Source: CAD feature listing. Evaluate the final solid. Frame: model axes, mm. A direction names the side the tool comes from. Give positions to 0.01 mm unless a question says otherwise; leave off trailing zeros. Write each loop counter-clockwise with the first axis right and the second up, starting at its lowest first coordinate (ties: lowest second). Pieces come first, ordered by that corner, then holes. Notation, with made-up numbers: (50.25, 17.25) -> (102.25, 17.25) arc R29 cw to (102.25, 51.25) -> close; hole circle Ø5 at (-13.5, 78). An arc over 180 degrees is marked (long way). Write item = value, one per line.
from build123d import *

# Parameters (mm, degrees)
BOSS_EXTRUDE1_DEPTH = 127
CUT_EXTRUDE1_REACH  = 39.846
SKETCH3_R           = 6.35


with BuildPart() as part:
    # Sketch1 → Boss-Extrude1 (new body, symmetric)
    with BuildSketch(Plane.XY):
        with BuildLine():
            Line((37.846, -38.1), (0, -38.1))
            Line((0, -38.1), (0, 38.1))
            Line((0, 38.1), (37.846, 38.1))
            Line((37.846, 38.1), (37.846, 38.095373852))
            Line((37.846, 38.095373852), (37.846, 38.07919906))
            ThreePointArc((37.846, 38.07919906), (37.304749426, 36.602159643), (35.937298827, 35.824550175))
            Line((35.937298827, 35.824550175), (12.279303519, 31.865559515))
            ThreePointArc((12.279303519, 31.865559515), (8.176951722, 29.532731112), (6.5532, 25.101612859))
            Line((6.5532, 25.101612859), (6.5532, -24.125928831))
            ThreePointArc((6.5532, -24.125928831), (8.176951722, -28.557047083), (12.279303519, -30.889875486))
            Line((12.279303519, -30.889875486), (35.725220919, -34.813376476))
            ThreePointArc((35.725220919, -34.813376476), (37.244610473, -35.677386996), (37.846, -37.318541904))
            Line((37.846, -37.318541904), (37.846, -38.1))
        make_face()
    extrude(amount=BOSS_EXTRUDE1_DEPTH, both=True)

    # Sketch3 → Cut-Extrude1 (cut, up to next)
    with BuildSketch(Plane.ZY, mode=Mode.PRIVATE) as cut_extrude1_sk1:
        with Locations((-15.875, 0)):
            Circle(SKETCH3_R)
    cut_extrude1_tool1 = extrude(cut_extrude1_sk1.sketch, amount=-CUT_EXTRUDE1_REACH, mode=Mode.PRIVATE) & part.part
    add(cut_extrude1_tool1.solids().sort_by_distance((0, 0, -15.875))[0], mode=Mode.SUBTRACT)
    # Sketch3 → Cut-Extrude1 (cut, up to next)
    with BuildSketch(Plane.ZY, mode=Mode.PRIVATE) as cut_extrude1_sk2:
        with Locations((15.875, 0)):
            Circle(SKETCH3_R)
    cut_extrude1_tool2 = extrude(cut_extrude1_sk2.sketch, amount=-CUT_EXTRUDE1_REACH, mode=Mode.PRIVATE) & part.part
    add(cut_extrude1_tool2.solids().sort_by_distance((0, 0, 15.875))[0], mode=Mode.SUBTRACT)


solid = part.part
1) Material intervals for L1, parallel to X at y = 1, z = 88.5; L2, parallel to Z at x = 2.5, y = -1.5; L3, parallel to Y at x = 24, z = 27.5, sorted ascending.
Computed:
L1 = 0 to 6.55
L2 = -127 to -22.05, -9.7 to 9.7, 22.05 to 127
L3 = -38.1 to -32.85, 33.83 to 38.1
2) Contact query for flat-ended pins moving along their axis: pin 1 (3 mm diameter, centred on y = 5.5, z = -10.5, fed in from -X); pin 2 (16.5 mm diameter, centred on y = 0, z = 15.875, fed in from +X). Output: stop coordinate, or through.
Computed:
pin_1 = 0
pin_2 = 6.55
3) Access query for faces 1 (the flat face through (0, -1, 2)), 2 (the flat face through (23.838, -32.824, 1.778)). Directions: +Z, -Z, +X, -X, +Y, -Y. A direction counts if a zero-diameter tool reaches every point of the face in a straight line with its end or side. Return the directions, or none.
Computed:
face_1 = +Z, -Z, -X, +Y, -Y
face_2 = +Z, -Z, +X
4) Cut plane A-A (y = 0). Return the cut outline in (x, z) (3 decimals).
Computed:
outline = (0, -127) -> (6.553, -127) -> (6.553, -22.225) -> (0, -22.225) -> close; (0, -9.525) -> (6.553, -9.525) -> (6.553, 9.525) -> (0, 9.525) -> close; (0, 22.225) -> (6.553, 22.225) -> (6.553, 127) -> (0, 127) -> close
5) Cut plane D-D (y = -15). Return the cut outline in (x, z), then the cut area to 3 significant figures.
Computed:
outline = (0, -127) -> (6.55, -127) -> (6.55, 127) -> (0, 127) -> close
area = 1,660 mm²
6) Draft query along Z for faces 3 (the cylindrical face through (3.23, 1.91, 21.93)), 4 (the flat face through (19, 38.1, 2)), 5 (the flat face through (6, 3, -127)). Return one class per face: pulls with the +Z half, pulls with the -Z half, needs draft (parallel to the pull), parting line crosses it, or undercut.
Computed:
face_3 = undercut
face_4 = needs draft
face_5 = pulls with the -Z half
7) Cut plane B-B (x = 23.5). Return the cut outline in (y, z).
Computed:
outline = (-38.1, -127) -> (-32.77, -127) -> (-32.77, 127) -> (-38.1, 127) -> close; (33.74, -127) -> (38.1, -127) -> (38.1, 127) -> (33.74, 127) -> close
